```python
from build123d import *

# Parameters (mm, degrees)
SKETCH1_W           = 348
SKETCH1_H           = 126
BOSS_EXTRUDE1_DEPTH = 20
SKETCH2_W           = 340
SKETCH2_H           = 118
CUT_EXTRUDE1_DEPTH  = 15
CUT_EXTRUDE2_REACH  = 217.759
CUT_EXTRUDE3_REACH  = 217.759
SKETCH5_W           = 20
SKETCH5_H           = 8
FILLET1_R           = 5


with BuildPart() as part:
    # Sketch1 → Boss-Extrude1 (new body)
    with BuildSketch(Plane.XY):
        Rectangle(SKETCH1_W, SKETCH1_H)
    extrude(amount=BOSS_EXTRUDE1_DEPTH)

    # Sketch2 → Cut-Extrude1 (cut)
    with BuildSketch(Plane.XY.offset(20)):
        Rectangle(SKETCH2_W, SKETCH2_H)
    extrude(amount=-CUT_EXTRUDE1_DEPTH, mode=Mode.SUBTRACT)

    # Sketch4 → Cut-Extrude2 (cut, up to next)
    with BuildSketch(Plane(origin=(0, 63, 0), x_dir=(1, 0, 0), z_dir=(0, 1, 0)), mode=Mode.PRIVATE) as cut_extrude2_sk1:
        with BuildLine():
            Line((122.39, -12.5), (137.39, -12.5))
            ThreePointArc((137.39, -12.5), (141.14, -16.25), (137.39, -20))
            Line((137.39, -20), (122.39, -20))
            ThreePointArc((122.39, -20), (118.64, -16.25), (122.39, -12.5))
        make_face()
    cut_extrude2_tool1 = extrude(cut_extrude2_sk1.sketch, amount=-CUT_EXTRUDE2_REACH, mode=Mode.PRIVATE) & part.part
    add(cut_extrude2_tool1.solids().sort_by_distance((129.89, 63, 16.25))[0], mode=Mode.SUBTRACT)

    # Sketch5 → Cut-Extrude3 (cut, up to next)
    with BuildSketch(Plane(origin=(0, 63, 0), x_dir=(1, 0, 0), z_dir=(0, 1, 0)), mode=Mode.PRIVATE) as cut_extrude3_sk1:
        with Locations((155.05, -14.81)):
            Rectangle(SKETCH5_W, SKETCH5_H)
    cut_extrude3_tool1 = extrude(cut_extrude3_sk1.sketch, amount=-CUT_EXTRUDE3_REACH, mode=Mode.PRIVATE) & part.part
    add(cut_extrude3_tool1.solids().sort_by_distance((155.05, 63, 14.81))[0], mode=Mode.SUBTRACT)

    # Fillet1
    fillet1_edges = [part.edges().sort_by_distance(p)[0] for p in [
        (-174, 63, 10),
        (174, 63, 10),
        (174, -63, 10),
        (-174, -63, 10),
    ]]
    fillet(fillet1_edges, radius=FILLET1_R)


solid = part.part
```
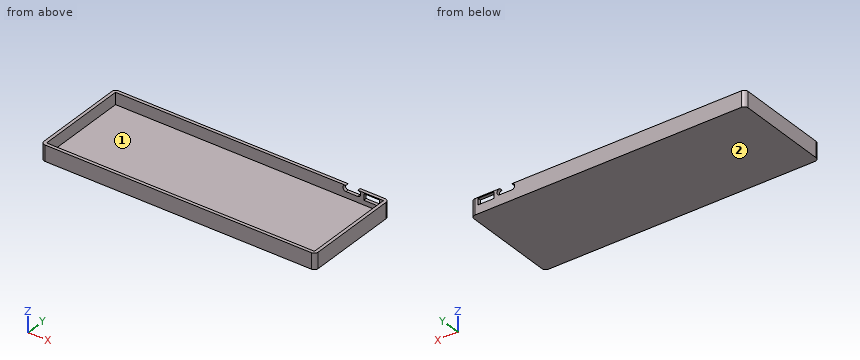
Verification items for the finished model (mm, model axes). Face numbers are marked on the shaded views. Coordinates: 2 decimals unless noted, no trailing zeros. Loops run counter-clockwise (first coordinate to the right, second up) from the corner with the lowest first, then second, coordinate; pieces in that order, holes last. Notation, with made-up numbers: (51.5, -12.5) - (105.5, -12.5) arc R27 ccw to (105.5, 9.5) - close; hole circle Ø2 at (53, 87.5). An arc over 180 degrees is marked (long way). Return JSON: item names as keys, results as strings.
1. Go/stop test with flat-tipped pins: pin 1 (1 mm diameter, centred on x = -59, y = 44, fed in from +Z); pin 2 (3 mm diameter, centred on y = 61.5, z = 15, fed in from -X); pin 3 (1.2 mm diameter, centred on y = 60.5, z = 16, fed in from +X). Record where each tip stops, or that it passes through.
Established:
{"pin 1": "stops at z = 5", "pin 2": "stops at x = -173.58", "pin 3": "stops at x = 173.62"}
2. Section check B-B, the plane y = -29. Record the boundary of the cut face in (x, z), then the cut area to 3 significant figures.
Established:
{"outline": "(-174, 0) - (174, 0) - (174, 20) - (170, 20) - (170, 5) - (-170, 5) - (-170, 20) - (-174, 20) - close", "area": "1,860 mm2"}
3. Section check A-A, the plane z = 15.5. Record the boundary of the cut face in (x, y), then the cut area to 3 significant figures.
Established:
{"outline": "(-174, -58) arc R5 ccw to (-169, -63) - (169, -63) arc R5 ccw to (174, -58) - (174, 58) arc R5 ccw to (169, 63) - (165.05, 63) - (165.05, 59) - (170, 59) - (170, -59) - (-170, -59) - (-170, 59) - (118.72, 59) - (118.72, 63) - (-169, 63) arc R5 ccw to (-174, 58) - close; (141.06, 59) - (145.05, 59) - (145.05, 63) - (141.06, 63) - close", "area": "3,540 mm2"}
4. Mould release check, pull along X, two halves, no side actions. Record for the marked faces 1 and 2: +X half, -X half, draft (parallel to the pull), parting line (faces both ways), or undercut.
Established:
{"face 1": "undercut", "face 2": "draft"}
5. Section check C-C, the plane x = -19. Record the boundary of the cut face in (y, z), then the cut area to 3 significant figures.
Established:
{"outline": "(-63, 0) - (63, 0) - (63, 20) - (59, 20) - (59, 5) - (-59, 5) - (-59, 20) - (-63, 20) - close", "area": "750 mm2"}
6. Thickness scan on L1, parallel to Y at x = 10.5, z = 11.5; L2, parallel to X at y = 11.5, z = 14.5; L3, parallel to Z at x = 115.5, y = 30. Record the ranges inside material, lowest first.
Established:
{"L1": "y = -63 to -59, 59 to 63", "L2": "x = -174 to -170, 170 to 174", "L3": "z = 0 to 5"}
